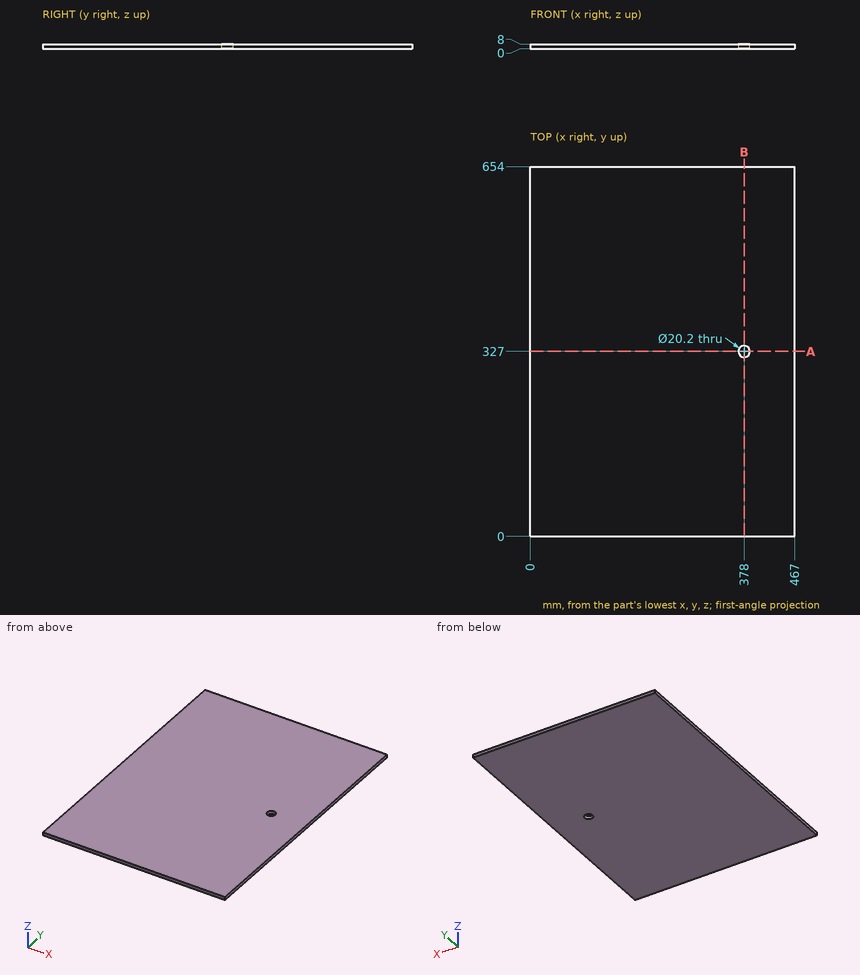
Could you check a few things on this drawing? It's one solid part, dimensions in mm from its lowest x, y, z. Round coordinates to 2 decimals unless told otherwise and drop trailing zeros. Write each loop counter-clockwise with the first axis right and the second up, starting at its lowest first coordinate (ties: lowest second). Pieces come first, ordered by that corner, then holes. Notation, with made-up numbers: (33, -30) -> (77, -30) arc R7 cw to (77, -18) -> close; hole circle Ø1 at (70.25, 38.25). An arc over 180 degrees is marked (long way). Use a Markdown table: item, result.
1. If we section it at B-B (x = 378): List the corners of the cut face in (y, z) for me.
Answer key:
| item | result |
|---|---|
| outline | (0, 0) -> (316.9, 0) -> (316.9, 8) -> (0, 8) -> close; (337.1, 0) -> (654, 0) -> (654, 8) -> (337.1, 8) -> close |
2. For pin 1 Ø1.5 at (x, z) = (188.5, 3.5) entering from -Y; pin 2 Ø16 at (x, y) = (378, 327) entering from +Z, each with a flat end and sliding along its axis, tell me the tip position at first contact or that it passes through.
Answer key:
| item | result |
|---|---|
| pin 1 | stops at y = 0 |
| pin 2 | passes through |
3. Please list where these lines run through material, in increasing order: probe 1 along X at (y, z) = (327, 2.75); probe 2 along Y at (x, z) = (378, 5.75).
Answer key:
| item | result |
|---|---|
| probe 1 | x = 0 to 367.9, 388.1 to 467 |
| probe 2 | y = 0 to 316.9, 337.1 to 654 |
4. If we section it at A-A (y = 327): List the corners of the cut face in (x, z) for me.
Answer key:
| item | result |
|---|---|
| outline | (0, 0) -> (367.9, 0) -> (367.9, 8) -> (0, 8) -> close; (388.1, 0) -> (467, 0) -> (467, 8) -> (388.1, 8) -> close |
